The listing builds one solid part. Answer for the finished solid, in the listing's coordinates (mm). A direction names the side the tool comes from. Coordinates: 2 decimals unless noted, no trailing zeros.
from build123d import *

# Parameters (mm, degrees)
CIRPATTERN1_COUNT = 2
CIRPATTERN1_ANGLE = 90
THDSCHPAT_COUNT   = 7
THDSCHPAT_PITCH   = 0.466666667


with BuildPart() as part:
    # BodySke → Base-Revolve (revolve)
    with BuildSketch(Plane.XY, mode=Mode.PRIVATE) as base_revolve_sk:
        with BuildLine():
            Line((0, 0), (5.727669073, 0))
            Line((5.727669073, 0), (5.727669073, 1.5))
            Line((5.727669073, 1.5), (2.427669073, 1.5))
            Line((2.427669073, 1.5), (1.177669073, 2.75))
            Line((1.177669073, 2.75), (0.529956332, 2.75))
            ThreePointArc((0.529956332, 2.75), (0.133696843, 1.400299407), (0, 0))
        make_face()
    revolve(base_revolve_sk.sketch.rotate(Axis((-15.875, 0, 0), (1, 0, 0)), 90), axis=Axis((-15.875, 0, 0), (1, 0, 0)))

    # Sketch3 → Cross section 0
    with BuildSketch(Plane(origin=(0, 0, 0), x_dir=(0, 0, -1), z_dir=(1, 0, 0))):
        with BuildLine():
            Line((0.415, -1.72), (-0.415, -1.72))
            Line((-0.415, -1.72), (-0.415, 1.72))
            Line((-0.415, 1.72), (0.415, 1.72))
            Line((0.415, 1.72), (0.415, -1.72))
        make_face()
    # Sketch4 → Cross section 1
    with BuildSketch(Plane(origin=(2.33, 0, 0), x_dir=(0, 0, -1), z_dir=(1, 0, 0))):
        with BuildLine():
            Line((0.2075, -0.2075), (-0.2075, -0.2075))
            Line((-0.2075, -0.2075), (-0.2075, 0.2075))
            Line((-0.2075, 0.2075), (0.2075, 0.2075))
            Line((0.2075, 0.2075), (0.2075, -0.2075))
        make_face()
    cross = loft(mode=Mode.SUBTRACT)

    # CirPattern1: Cross ×2 about axis
    cirpattern1_axis = Axis((0, 0, 0), (1, 0, 0))
    for i in range(1, CIRPATTERN1_COUNT):
        add(cross.rotate(cirpattern1_axis, i * CIRPATTERN1_ANGLE / (CIRPATTERN1_COUNT - 1)), mode=Mode.SUBTRACT)

    # ThdSchSke → ThreadSchematic (revolve, cut)
    with BuildSketch(Plane.XY):
        Polygon((2.927669073, -1.2195), (2.731260858, -1.5), (2.731260858, -1.875), (3.124077287, -1.875), (3.124077287, -1.5), align=None)
    threadschematic = revolve(axis=Axis((-3.175, 0, 0), (1, 0, 0)), mode=Mode.SUBTRACT)

    # ThdSchPat: ThreadSchematic ×7
    with Locations(*[(i * THDSCHPAT_PITCH, 0, 0) for i in range(1, THDSCHPAT_COUNT)]):
        add(threadschematic, mode=Mode.SUBTRACT)


solid = part.part
1. Find the intervals of material crossed by L1, parallel to Z at x = 0.75, y = 0.95; L2, parallel to Y at x = 0.65, z = -0.2; L3, parallel to X at y = -1.05, z = 0.15, in increasing order.
Results found:
L1: z = -2.58 to -0.35, 0.35 to 2.58
L2: y = -2.74 to -1.3, 1.3 to 2.74
L3: x = 1.03 to 5.73
2. Flat-ended cylindrical pins translate along their axes: P1, Ø3, axis at x = 3.5, y = -2, coming from the +Z side; P2, Ø0.5, axis at y = 0, z = 0, coming from the -X side; P3, Ø1, axis at y = 2, z = -0.5, coming from the +X side. Find the tip coordinate at first contact, or state that the pin passes through.
Results found:
P1: stops at z = 1.41
P2: stops at x = 2.26
P3: stops at x = 2.37
3. A tool of negligible diameter and unlimited length cuts with its end or side. For faces 1 (the cylindrical face through (0.849, 2.685, -0.596)), 2 (the cylindrical face through (2.58, -0.45, 1.43)), from which of +Z, -Z, +X, -X, +Y, -Y can it reach the whole face along a straight path? Write none if from no direction.
Results found:
face 1: +X, -X
face 2: +X
